```python
from build123d import *

# Parameters (mm, degrees)
ESQUISSE1_W             = 400
ESQUISSE1_H             = 200
BOSS_EXTRU_1_DEPTH      = 6
ESQUISSE2_R             = 2.5
ENL_V_MAT_EXTRU_1_DEPTH = 224.687281713
ESQUISSE3_R             = 4.5
ENL_V_MAT_EXTRU_2_DEPTH = 224.687281713


with BuildPart() as part:
    # Esquisse1 → Boss.-Extru.1 (new body)
    with BuildSketch(Plane(origin=(0, 0, 0), x_dir=(1, 0, 0), z_dir=(0, 1, 0))):
        Rectangle(ESQUISSE1_W, ESQUISSE1_H)
    extrude(amount=BOSS_EXTRU_1_DEPTH)

    # Esquisse2 → Enlèv. mat.-Extru.1 (cut, through all)
    with BuildSketch(Plane(origin=(0, 6, 0), x_dir=(1, 0, 0), z_dir=(0, 1, 0))):
        with Locations(Location((-100, 76, 0), (0, 0, 270))):
            Circle(ESQUISSE2_R)
        with Locations(Location((100, 76, 0), (0, 0, 270))):
            Circle(ESQUISSE2_R)
        with Locations(Location((100, -76, 0), (0, 0, 270))):
            Circle(ESQUISSE2_R)
        with Locations(Location((-100, -76, 0), (0, 0, 270))):
            Circle(ESQUISSE2_R)
        with Locations(Location((-176, 40, 0), (0, 0, 270))):
            Circle(ESQUISSE2_R)
        with Locations(Location((-176, -40, 0), (0, 0, 270))):
            Circle(ESQUISSE2_R)
        with Locations(Location((176, -40, 0), (0, 0, 270))):
            Circle(ESQUISSE2_R)
        with Locations(Location((176, 40, 0), (0, 0, 270))):
            Circle(ESQUISSE2_R)
    extrude(amount=-ENL_V_MAT_EXTRU_1_DEPTH, mode=Mode.SUBTRACT)

    # Esquisse3 → Enlèv. mat.-Extru.2 (cut, through all)
    with BuildSketch(Plane(origin=(0, 6, 0), x_dir=(1, 0, 0), z_dir=(0, 1, 0))):
        with Locations(Location((0, -76, 0), (0, 0, 270))):
            Circle(ESQUISSE3_R)
    extrude(amount=-ENL_V_MAT_EXTRU_2_DEPTH, mode=Mode.SUBTRACT)


solid = part.part
```
Input: part model. Units: mm. Frame: model coordinates. Give positions to 0.01 mm unless a question says otherwise; leave off trailing zeros. Order: outer loops, then holes, each group sorted by start corner. A loop starts at its lowest first (then second) coordinate and runs counter-clockwise, first axis right, second up.
1. Pin query (flat end, axial travel): pin 1 (4.5 mm diameter, centred on x = 100, z = 76, fed in from +Y). Return the tip coordinate at first contact, or that it passes through.
Derived:
pin 1: passes through
2. Material intervals for L1, parallel to Z at x = 176, y = 3.9; L2, parallel to X at y = 2, z = -40; L3, parallel to X at y = 4.25, z = 76, sorted ascending.
Derived:
L1: z = -100 to -42.5, -37.5 to 37.5, 42.5 to 100
L2: x = -200 to -178.5, -173.5 to 173.5, 178.5 to 200
L3: x = -200 to -102.5, -97.5 to -4.5, 4.5 to 97.5, 102.5 to 200
3. Mould query, pull axis X, two halves, no side actions, for faces 1 (the cylindrical face through (-1.72, 3.04, 80.16)), 2 (the flat face through (-3, 6, -1)). Classes: released by +X, released by -X, zero draft, split by the parting line, or undercut.
Derived:
face 1: undercut
face 2: zero draft
4. Section A-A on x = 0. Return the cut outline in (y, z).
Derived:
outline: (0, -100) - (6, -100) - (6, 71.5) - (0, 71.5) - close; (0, 80.5) - (6, 80.5) - (6, 100) - (0, 100) - close
